Read the model definition and answer for the solid it produces. Units are mm, in the model's axes. Face numbers are marked on the shaded views. Coordinates: 2 decimals unless noted, no trailing zeros. Put each result on its own line as item: value.
from build123d import *

# Parameters (mm, degrees)
BOSS_EXTRUDE1_DEPTH  = 6
BOSS_EXTRUDE2_DEPTH  = 2
BOSS_EXTRUDE2_TAPER  = 30
SKETCH6_R            = 6
BOSS_EXTRUDE3_DEPTH  = 1
SKETCH7_R            = 6
CUT_EXTRUDE1_DEPTH   = 3
FILLET1_START        = -1
FILLET1_DEPTH        = 4
CHAMFER1_SIZE        = 1
M4_CLEARANCE_HOLE1_D = 4.5


with BuildPart() as part:
    # Sketch1 → Boss-Extrude1 (new body)
    with BuildSketch(Plane.XY):
        with BuildLine():
            ThreePointArc((-5.731715344, -1.774102368), (-1.774102368, 5.731715344), (5.731715344, 1.774102368))
            add(Edge.make_bspline(
                [(5.731715344, 1.774102368), (5.862890335, 1.350306246), (6.10195439, 0.511836894), (6.5513215, -1.302172264), (7.055062132, -3.775725238), (7.600837363, -7.119895561), (8.261344969, -12.065805628), (8.9758633, -19.127681627), (9.671419516, -28.81644754), (10.210024516, -39.49120604), (10.721813898, -54.718080156), (10.977124068, -75), (10.721813898, -95.281919844), (10.210024516, -110.50879396), (9.671419516, -121.18355246), (8.9758633, -130.872318373), (8.261344969, -137.934194372), (7.600837363, -142.880104439), (7.055062132, -146.224274762), (6.5513215, -148.697827736), (6.10195439, -150.511836894), (5.862890335, -151.350306246), (5.731715344, -151.774102368)],
                knots=[0, 0, 0, 0, 0.015625, 0.03125, 0.0625, 0.09375, 0.125, 0.1875, 0.25, 0.3125, 0.375, 0.5, 0.625, 0.6875, 0.75, 0.8125, 0.875, 0.90625, 0.9375, 0.96875, 0.984375, 1, 1, 1, 1], degree=3))
            ThreePointArc((5.731715344, -151.774102368), (-1.774102368, -155.731715344), (-5.731715344, -148.225897632))
            add(Edge.make_bspline(
                [(-5.731715344, -1.774102368), (-5.692087495, -1.902130803), (-5.618775496, -2.148725819), (-5.458728189, -2.727966614), (-5.255155063, -3.54817606), (-5.006643591, -4.688807627), (-4.677115643, -6.39564749), (-4.27454567, -8.85601244), (-3.817957958, -12.269624912), (-3.392734432, -16.09709888), (-2.871156001, -21.69677536), (-2.308115125, -29.531273979), (-1.780341203, -39.985350621), (-1.402466695, -51.223362083), (-1.175470707, -62.981825406), (-1.099764647, -75), (-1.175470707, -87.018174594), (-1.402466695, -98.776637917), (-1.780341203, -110.014649379), (-2.308115125, -120.468726021), (-2.871156001, -128.30322464), (-3.392734432, -133.90290112), (-3.817957958, -137.730375088), (-4.27454567, -141.14398756), (-4.677115643, -143.60435251), (-5.006643591, -145.311192373), (-5.255155063, -146.45182394), (-5.458728189, -147.272033386), (-5.618775496, -147.851274181), (-5.692087495, -148.097869197), (-5.731715344, -148.225897632)],
                knots=[0, 0, 0, 0, 0.0078125, 0.015625, 0.03125, 0.046875, 0.0625, 0.09375, 0.125, 0.15625, 0.1875, 0.25, 0.3125, 0.375, 0.4375, 0.5, 0.5625, 0.625, 0.6875, 0.75, 0.8125, 0.84375, 0.875, 0.90625, 0.9375, 0.953125, 0.96875, 0.984375, 0.9921875, 1, 1, 1, 1], degree=3))
        make_face()
    extrude(amount=BOSS_EXTRUDE1_DEPTH)

    # Sketch2 → Boss-Extrude2 (add)
    with BuildSketch(Plane.XY.offset(6)):
        with BuildLine():
            add(Edge.make_bspline(
                [(3.842779218, -144.149098541), (3.99518889, -143.228609095), (4.133577932, -142.306808915), (4.482341024, -139.816291581), (4.674300588, -138.24585293), (5.022834622, -135.101667614), (5.179034802, -133.527885959), (5.608568883, -128.802888823), (5.843693204, -125.648101279), (6.249577099, -119.332508984), (6.419662658, -116.171641222), (6.857535334, -106.68227104), (7.05432563, -100.34499664), (7.313633365, -87.672679841), (7.436364195, -75.000225736), (7.313637964, -62.327524864), (7.05431874, -49.65468667), (6.857549017, -43.318319211), (6.419745963, -33.830017305), (6.249687473, -30.669449522), (5.843863318, -24.354304808), (5.608771942, -21.1996664), (5.179285888, -16.474715495), (5.023101498, -14.900919175), (4.67459471, -11.756621418), (4.482646895, -10.186085829), (4.133804085, -7.694692501), (3.995316322, -6.772156482), (3.842779302, -5.850901403)],
                knots=[0.044109896, 0.044109896, 0.044109896, 0.044109896, 0.0625, 0.0625, 0.09375, 0.09375, 0.125, 0.125, 0.1875, 0.1875, 0.25, 0.25, 0.375, 0.375, 0.5, 0.625, 0.625, 0.75, 0.75, 0.8125, 0.8125, 0.875, 0.875, 0.90625, 0.90625, 0.9375, 0.9375, 0.955902495, 0.955902495, 0.955902495, 0.955902495], degree=3))
            ThreePointArc((3.842779302, -5.850901403), (1.496097545, -6.838252126), (-1.048489728, -6.921030941))
            add(Edge.make_bspline(
                [(-1.048489728, -6.921030941), (-0.887726028, -7.908676873), (-0.743269436, -8.898495118), (-0.400727329, -11.426505037), (-0.218072452, -12.966752267), (0.114129955, -16.051657047), (0.263395019, -17.596352224), (0.674511995, -22.235323757), (0.900378843, -25.335536499), (1.290535741, -31.537230608), (1.454172696, -34.639030666), (1.875705513, -43.946533714), (2.065405192, -50.154303756), (2.315616461, -62.573759578), (2.374993429, -68.785688578), (2.37500657, -81.21228644), (2.315647979, -87.424382498), (2.065406806, -99.845909639), (1.875647227, -106.055756994), (1.453897372, -115.3665461), (1.290239744, -118.467676771), (0.900441737, -124.663261276), (0.675011926, -127.757791041), (0.264495235, -132.3918521), (0.115436706, -133.935233344), (-0.216369082, -137.018395892), (-0.398831003, -138.558207687), (-0.741756199, -141.091163775), (-0.886846381, -142.085950818), (-1.048489537, -143.07896903)],
                knots=[0.042345585, 0.042345585, 0.042345585, 0.042345585, 0.0625, 0.0625, 0.09375, 0.09375, 0.125, 0.125, 0.1875, 0.1875, 0.25, 0.25, 0.375, 0.375, 0.5, 0.5, 0.625, 0.625, 0.75, 0.75, 0.8125, 0.8125, 0.875, 0.875, 0.90625, 0.90625, 0.9375, 0.9375, 0.957747168, 0.957747168, 0.957747168, 0.957747168], degree=3))
            ThreePointArc((-1.048489537, -143.07896903), (1.49609759, -143.161747884), (3.842779218, -144.149098541))
        make_face()
    extrude(amount=BOSS_EXTRUDE2_DEPTH, taper=BOSS_EXTRUDE2_TAPER)

    # Sketch5 → Cut-Revolve1 (revolve, cut)
    with BuildSketch(Plane(origin=(0, 0, 0), x_dir=(0, 0, -1), z_dir=(1, 0, 0))):
        with BuildLine():
            ThreePointArc((-6, -140.397478747), (-6.513167019, -137.235201087), (-8, -134.397478747))
            Line((-8, -134.397478747), (-8, -142.397478747))
            Line((-8, -142.397478747), (-6, -144.149098541))
            Line((-6, -144.149098541), (-6, -140.397478747))
        make_face()
    revolve(axis=Axis((0, -150, 0), (0, 0, 1)), mode=Mode.SUBTRACT)

    # Sketch5<4> → Cut-Revolve2 (revolve, cut)
    with BuildSketch(Plane(origin=(0, 0, 0), x_dir=(0, 0, -1), z_dir=(1, 0, 0))):
        with BuildLine():
            Line((-8, -7.602521037), (-6, -5.850901403))
            ThreePointArc((-6, -5.850901403), (-6.513167019, -9.013179064), (-8, -11.850901403))
            Line((-8, -11.850901403), (-8, -7.602521037))
        make_face()
    revolve(axis=Axis((0, 0, 0), (0, 0, 1)), mode=Mode.SUBTRACT)

    # Sketch6 → Boss-Extrude3 (add)
    with BuildSketch(Plane.XY.offset(6)):
        with Locations(Location((0, 0, 0), (0, 0, 197.19854122))):
            Circle(SKETCH6_R)
    extrude(amount=BOSS_EXTRUDE3_DEPTH)

    # Sketch7 → Cut-Extrude1 (cut)
    with BuildSketch(Plane(origin=(0, 0, 0), x_dir=(-1, 0, 0), z_dir=(0, 0, -1))):
        with Locations(Location((0, 0, 0), (0, 0, 342.80145878))):
            Circle(SKETCH7_R)
    extrude(amount=-CUT_EXTRUDE1_DEPTH, mode=Mode.SUBTRACT)

    # Fillet1: read off the stored shape, not the designer's step
    # Fillet1 outline → Fillet1 (cut)
    with BuildSketch(Plane.XY.offset(FILLET1_START)):
        with BuildLine():
            add(Edge.make_bspline(
                [(-5.731715344, -1.774102368), (-5.692087495, -1.902130803), (-5.618775496, -2.148725819), (-5.458728189, -2.727966614), (-5.255155063, -3.54817606), (-5.006643591, -4.688807627), (-4.777507184, -5.875654311), (-4.632728696, -6.704930928), (-4.56971799, -7.081374578)],
                knots=[0, 0, 0, 0, 0.0078125, 0.015625, 0.03125, 0.046875, 0.0625, 0.074709213, 0.074709213, 0.074709213, 0.074709213], degree=3))
            ThreePointArc((-4.56971799, -7.081374578), (-4.005198612, -5.645063514), (-2.472239677, -5.466994694))
            ThreePointArc((-2.472239677, -5.466994694), (-4.498397818, -3.970442931), (-5.731715344, -1.774102368))
        make_face()
        with BuildLine():
            ThreePointArc((5.731715344, 1.774102368), (5.876589294, -1.210660261), (4.563775855, -3.895118733))
            ThreePointArc((4.563775855, -3.895118733), (6.101473007, -3.422320762), (7.182806929, -4.613440991))
            add(Edge.make_bspline(
                [(5.731715344, 1.774102368), (5.862890335, 1.350306246), (6.10195439, 0.511836894), (6.5513215, -1.302172264), (6.902345222, -3.025828681), (7.137523842, -4.351431198), (7.182806929, -4.613440991)],
                knots=[0, 0, 0, 0, 0.015625, 0.03125, 0.0625, 0.070065175, 0.070065175, 0.070065175, 0.070065175], degree=3))
        make_face()
    extrude(amount=FILLET1_DEPTH, mode=Mode.SUBTRACT)

    # Chamfer1
    chamfer1_edges = [part.edges().sort_by_distance(p)[0] for p in [
        (-1.128874241, -77.718314318, 0),
        (-1.774102368, -155.731715344, 0),
        (10.869440998, -78.27732173, 0),
        (-4.005198612, -5.645063514, 0),
        (1.308177895, -5.855652875, 0),
        (6.101473007, -3.422320762, 0),
    ]]
    chamfer(chamfer1_edges, length=CHAMFER1_SIZE)

    # M4 Clearance Hole1 (through all)
    with Locations(Plane.XY.offset(7)):
        with Locations((0, 0), (0, -150)):
            Hole(M4_CLEARANCE_HOLE1_D / 2)


solid = part.part
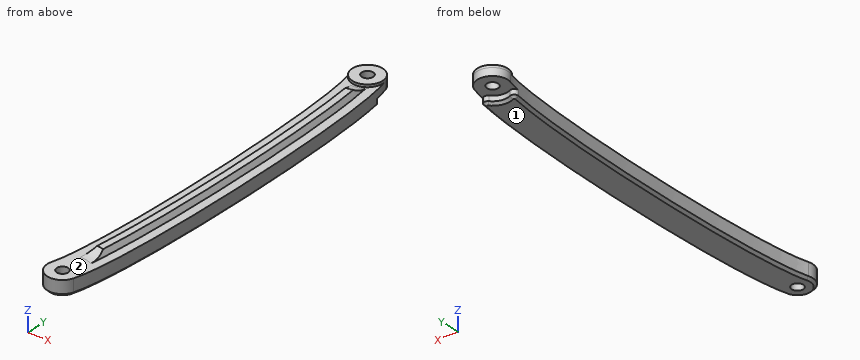
Q1. For a pull along Y with two mould halves and no side action, classify the marked faces 1 and 2 as +Y half, -Y half, draft (parallel to the pull), parting line (faces both ways), or undercut.
Answers below:
face 1: draft
face 2: undercut
Q2. Given pin 1 (6.5 mm diameter, centred on x = 0, y = -3.5, fed in from -Z); pin 2 (4 mm diameter, centred on x = -3, z = 2.5, fed in from +Y) (3 decimals); pin 3 (6 mm diameter, centred on x = -1.5, y = -0.5, fed in from +Z), each flat-ended and moving along its own axis, determine where each tip first touches the part or whether it passes through.
Answers below:
pin 1: stops at z = 0.25
pin 2: stops at y = 5.905
pin 3: stops at z = 7
Q3. Consider line 1 along Y through (x, z) = (0, 3.9); line 2 along Y through (x, z) = (1.25, 5); line 3 along Z through (x, y) = (8.75, -67.5). Determine where each line is inside the solid, lowest interval first.
Answers below:
line 1: y = -156 to -152.25, -147.75 to -2.25, 2.25 to 6
line 2: y = -155.87 to -151.87, -148.13 to -1.87, 1.87 to 5.87
line 3: z = 0 to 6
